Design review of the part shown in the three views and the two pictorial views. Dimensions are in mm from the part's minimum x, y and z. Coordinates: 2 decimals unless noted, no trailing zeros. Loops run counter-clockwise (first coordinate to the right, second up) from the corner with the lowest first, then second, coordinate; pieces in that order, holes last. Notation, with made-up numbers: (-35.75, -20.5) - (8.25, -20.5) arc R15 cw to (8.25, 4.5) - close; hole circle Ø11 at (17, 17.25). An arc over 180 degrees is marked (long way). One line per question, with ' | ' between items.
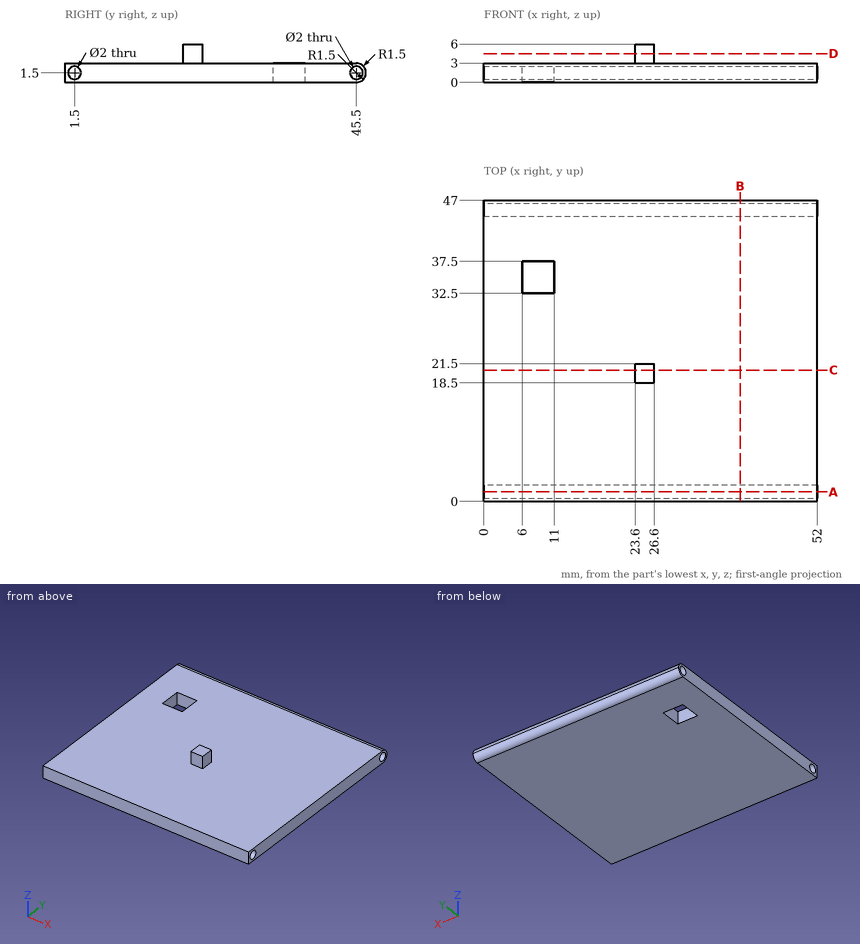
Q1. Take a section at B-B (x = 40). State how many separate pieces and enclosed holes the cut face has, plus the area to 3 significant figures.
Returned:
separate pieces: 1 | enclosed holes: 2 | area: 134 mm²
Q2. Take a section at A-A (y = 1.5). Give the boundary of the cut face in (x, z), plus the area to 3 significant figures.
Returned:
outline: (0, 0) - (52, 0) - (52, 0.5) - (0, 0.5) - close; (0, 2.5) - (52, 2.5) - (52, 3) - (0, 3) - close | area: 52.0 mm²
Q3. For pin 1 (1.8 mm diameter, centred on y = 1.5, z = 1.5, fed in from -X); pin 2 (2.5 mm diameter, centred on x = 25.5, z = 4.5, fed in from -Y); pin 3 (0.9 mm diameter, centred on y = 20, z = 4.5, fed in from +X); pin 4 (3.5 mm diameter, centred on x = 24.5, z = 4.5, fed in from +Y), all flat-tipped, find the tip position at first contact; note any pin that passes through.
Returned:
pin 1: passes through | pin 2: stops at y = 18.5 | pin 3: stops at x = 26.6 | pin 4: stops at y = 46.33
Q4. Take a section at D-D (z = 4.5). Give the boundary of the cut face in (x, y).
Returned:
outline: (23.6, 18.5) - (26.6, 18.5) - (26.6, 21.5) - (23.6, 21.5) - close
Q5. To check wall thickness, follow line 1 along Z through (x, y) = (11.5, 1.5); line 2 along Z through (x, y) = (47, 15); line 3 along Z through (x, y) = (38, 45). State the ranges of each line that lie inside material, in increasing order.
Returned:
line 1: z = 0 to 0.5, 2.5 to 3 | line 2: z = 0 to 3 | line 3: z = 0 to 0.63, 2.37 to 3
Q6. Take a section at C-C (y = 20.5). Give the boundary of the cut face in (x, z), plus the area to 3 significant figures.
Returned:
outline: (0, 0) - (52, 0) - (52, 3) - (26.6, 3) - (26.6, 6) - (23.6, 6) - (23.6, 3) - (0, 3) - close | area: 165 mm²
